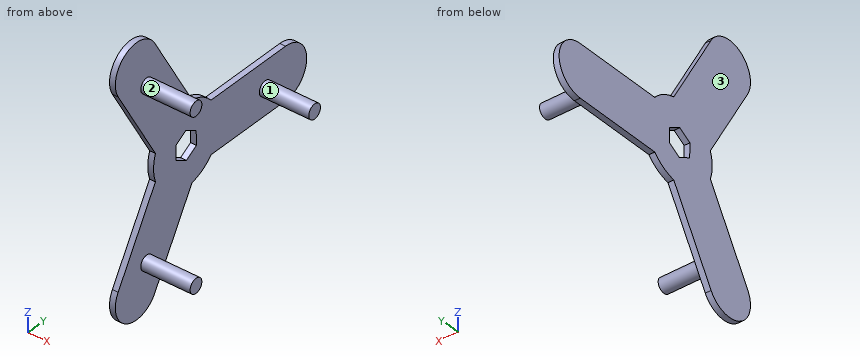
Autodesk Inventor part; units mm, degrees
ref_plane "YZ Plane" through (0, 0, 0) normal (1, 0, 0) x (0, 1, 0)
ref_plane "XZ Plane" through (0, 0, 0) normal (0, 1, 0) x (-1, 0, 0)
ref_plane "XY Plane" through (0, 0, 0) normal (0, 0, 1) x (1, 0, 0)
sketch "Esboço1" plane through (0, 0, 0) normal (1, 0, 0) x (0, 1, 0)
  circle A0 centre (0, 0) radius 51.5625
  dimension "d0" = 103.125
extrude "Extrusão1" add sketch "Esboço1" along normal blind 2
sketch "Esboço2" plane through (2, 0, 0) normal (1, 0, 0) x (0, 0, -1)
  point P0 (0, 0)
sketch "Esboço3" plane through (2, 0, 0) normal (1, 0, 0) x (0, 0, -1)
  line L0 (-44.5522, -25.7222) -> (-12.0542, -6.9595)
  line L1 (12.0542, -6.9595) -> (44.5522, -25.7222)
  line L2 (0, 13.919) -> (0, 51.4445)
  circle A0 centre (0, 0) radius 51.4445
  circle A1 centre (0, 0) radius 33.75
  circle A2 centre (0, 0) radius 51.5625
  line L3 (-44.5522, -25.7222) -> (0, 0) construction
  line L4 (-32.2394, -29.0214) -> (-4.6786, -13.1092)
  line L5 (-13.6921, 2.5028) -> (-41.253, -13.4095)
  arc A3 (-41.253, -13.4095) -> (-32.2394, -29.0214) centre (-36.7462, -21.2154) ccw
  line L6 (0, 13.919) -> (0, 51.4445)
  line L7 (0, 0) -> (0, 51.4445) construction
  line L8 (9.0136, 10.6063) -> (9.0136, 42.4309)
  line L9 (-9.0136, 42.4309) -> (-9.0136, 10.6063)
  arc A4 (9.0136, 42.4309) -> (-9.0136, 42.4309) centre (0, 42.4309) ccw
  line L10 (12.0542, -6.9595) -> (44.5522, -25.7222)
  line L11 (0, 0) -> (44.5522, -25.7222) construction
  line L12 (4.6786, -13.1092) -> (32.2394, -29.0214)
  line L13 (41.253, -13.4095) -> (13.6921, 2.5028)
  arc A5 (32.2394, -29.0214) -> (41.253, -13.4095) centre (36.7462, -21.2154) ccw
  arc A6 (-9.0136, 10.6063) -> (-13.6921, 2.5028) centre (0, 0) ccw
  arc A7 (-4.6786, -13.1092) -> (4.6786, -13.1092) centre (0, 0) ccw
  arc A8 (13.6921, 2.5028) -> (9.0136, 10.6063) centre (0, 0) ccw
  circle A9 centre (0, 33.75) radius 2.5
  circle A10 centre (29.2284, -16.875) radius 2.5
  circle A11 centre (-29.2284, -16.875) radius 2.5
  point P0 (-22.2761, -12.8611)
  point P1 (0, 51.4445)
  point P2 (0, 25.7222)
  point P3 (44.5522, -25.7222)
  point P4 (22.2761, -12.8611)
  dimension "d5" = 5
  dimension "d6" = 5
  dimension "d7" = 5
  dimension "d8" = 103.125
  dimension "d9" = 67.5
extrude "Extrusão2" cut sketch "Esboço3" against normal blind 2 contours A3 L5 A1 A11 L0 | L0 A11 A1 L4 A3 | A11 A1 L0 | L0 A1 A11 | A4 L8 A1 A9 L2 | L2 A9 A1 L9 A4 | A5 L12 A1 A10 L1 | L1 A10 A1 L13 A5 | A1 A11 L0 | L0 A11 A1 | A1 L5 A6 L9 A9 L8 A8 L13 A10 L12 A7 L4 A11 | A9 A1 L2 | L2 A1 A9 | A10 A1 L1 | L1 A1 A10 | A1 A9 L2 | L2 A9 A1 | A1 A10 L1 | L1 A10 A1 keep common part
sketch "Esboço4" plane through (2, 0, 0) normal (1, 0, 0) x (0, 0, -1)
  circle A0 centre (0, 0) radius 33.75
  circle A1 centre (0, 33.75) radius 2.5
  circle A2 centre (-29.2284, -16.875) radius 2.5
  circle A3 centre (29.2284, -16.875) radius 2.5
  dimension "d10" = 67.5
  dimension "d11" = 5
  dimension "d14" = 360
extrude "Extrusão3" add sketch "Esboço4" along normal blind 17 contours A1 A0 | A0 A1 | A3 A0 | A0 A3 | A2 A0 | A0 A2
sketch "Esboço5" plane through (0, 0, 0) normal (-1, 0, 0) x (0, 0, 1)
  line L0 (5, -0.0957) -> (2.4171, -4.378)
  line L1 (2.4171, -4.378) -> (-2.5829, -4.2823)
  line L2 (-2.5829, -4.2823) -> (-5, 0.0957)
  line L3 (-5, 0.0957) -> (-2.4171, 4.378)
  line L4 (-2.4171, 4.378) -> (2.5829, 4.2823)
  line L5 (2.5829, 4.2823) -> (5, -0.0957)
  point P0 (0, 0)
  dimension "d18" = 10
extrude "Extrusão4" cut sketch "Esboço5" against normal blind 17
equation "\"d5\" = D_Furo_Planeta"
equation "\"d6\" = D_Furo_Planeta"
equation "\"d7\" = D_Furo_Planeta"
equation "\"d11\" = D_Furo_Planeta"
equation "\"modulo\" = 1.5"
equation "\"delta\" = 0.3"
equation "\"D_Furo_Sol\" = 8"
equation "\"D_Furo_Planeta\" = 5"
equation "\"Rendimento_eta\" = 0.85"
equation "\"Teste_Montagem\" = 0"
properties part number "Porta_Satelite"
The listing builds one solid part. Answer for the finished solid, in the listing's coordinates (mm). Face numbers are marked on the shaded views. Coordinates: 2 decimals unless noted, no trailing zeros. Write each loop counter-clockwise with the first axis right and the second up, starting at its lowest first coordinate (ties: lowest second). Pieces come first, ordered by that corner, then holes. Notation, with made-up numbers: (50, 89) - (91, 89) arc R31 cw to (91, 128) - close; hole circle Ø8 at (-38, 29). An arc over 180 degrees is marked (long way). Return JSON: item names as keys, results as strings. Group by question number.
Q1. The part is cut by section C-C on x = 17. Write down the section's boundary in (y, z) (3 decimals).
Q2. The part is cut by section A-A on y = -3. Write down the section's boundary in (x, z), and give its area (3 significant figures).
Q3. The part is cut by section D-D on y = 33.75. Write down the section's boundary in (x, z).
Q4. Find the intervals of material crossed by line 1 along X through (y, z) = (-8, 12.5); line 2 along Y through (x, z) = (1.5, -21.5); line 3 along Y through (x, z) = (11, 28), in increasing order. Write a range as [from, to].
Q5. The part is cut by section B-B on z = 0. Write down the section's boundary in (x, y).
Q6. Flat-ended cylindrical pins translate along their axes: pin 1 Ø0.6 at (x, y) = (0.5, 21.5) entering from -Z; pin 2 Ø3 at (x, y) = (16.5, 28.5) entering from +Z; pin 3 Ø3 at (x, z) = (14.5, 28) entering from +Y (3 decimals); pin 4 Ø2 at (x, y) = (4.5, -19.5) entering from -Z. Find the tip coordinate at first contact, or state that the pin passes through.
Q7. For a pull along Z with two mould halves and no side action, classify the marked faces 1, 2 and 3 as +Z half, -Z half, draft (parallel to the pull), parting line (faces both ways), or undercut.
Evaluation:
{
 "1": {"outline": "circle Ø5 at (-16.875, -29.228); circle Ø5 at (-16.875, 29.228); circle Ø5 at (33.75, 0)"},
 "2": {"outline": "(0, -23.22) - (2, -23.22) - (2, -3.29) - (0, -3.29) - close; (0, 3.25) - (2, 3.25) - (2, 23.22) - (0, 23.22) - close", "area": "79.8 mm2"},
 "3": {"outline": "(0, -9.01) - (2, -9.01) - (2, -2.5) - (19, -2.5) - (19, 2.5) - (2, 2.5) - (2, 9.01) - (0, 9.01) - close"},
 "4": {"line 1": "x = [0, 2]", "line 2": "y = [-22.82, -2.01]", "line 3": "y = [-19.05, -14.7]"},
 "5": {"outline": "(0, -13.92) - (2, -13.92) - (2, -4.33) - (0, -4.33) - close; (0, 4.33) - (2, 4.33) - (2, 31.25) - (19, 31.25) - (19, 36.25) - (2, 36.25) - (2, 51.44) - (0, 51.44) - close"},
 "6": {"pin 1": "stops at z = -9.01", "pin 2": "passes through", "pin 3": "stops at y = -14.375", "pin 4": "stops at z = -31.13"},
 "7": {"face 1": "parting line", "face 2": "undercut", "face 3": "draft"}
}
